```python
from build123d import *

# Parameters (mm, degrees)
SKETCH1_W           = 15
SKETCH1_H           = 35
SKETCH1_W_2         = 1.272906456
SKETCH1_H_2         = 13.426112712
SKETCH1_R           = 1.6
BOSS_EXTRUDE4_DEPTH = 10
SKETCH1_9_R         = 2.4
SKETCH1_9_R_2       = 1.6
CUT_EXTRUDE3_DEPTH  = 8
SKETCH1_10_W        = 15
SKETCH1_10_H        = 5
SKETCH1_10_W_2      = 5
BOSS_EXTRUDE5_DEPTH = 13
BOSS_EXTRUDE6_START = 13
SKETCH1_11_W        = 5
SKETCH1_11_H        = 5
SKETCH1_11_W_2      = 15
BOSS_EXTRUDE6_DEPTH = 10


with BuildPart() as part:
    # Sketch1 → Boss-Extrude4 (new body)
    with BuildSketch(Plane.XY):
        Rectangle(SKETCH1_W, SKETCH1_H)
        with Locations((0, 9.851749103)):
            Rectangle(SKETCH1_W_2, SKETCH1_H_2, mode=Mode.SUBTRACT)
        Circle(SKETCH1_R, mode=Mode.SUBTRACT)
    extrude(amount=BOSS_EXTRUDE4_DEPTH)

    # Sketch1_9 → Cut-Extrude3 (cut)
    with BuildSketch(Plane.XY):
        Circle(SKETCH1_9_R)
        Circle(SKETCH1_9_R_2, mode=Mode.SUBTRACT)
    extrude(amount=CUT_EXTRUDE3_DEPTH, mode=Mode.SUBTRACT)

    # Sketch1_10 → Boss-Extrude5 (add)
    with BuildSketch(Plane.XY):
        with Locations((0, -15)):
            Rectangle(SKETCH1_10_W, SKETCH1_10_H)
        with Locations((-5, 15)):
            Rectangle(SKETCH1_10_W_2, SKETCH1_10_H)
        with Locations((5, 15)):
            Rectangle(SKETCH1_10_W_2, SKETCH1_10_H)
    extrude(amount=BOSS_EXTRUDE5_DEPTH)

    # Sketch1_11 → Boss-Extrude6 (add)
    # profile 1 of 4: a face of its own
    with BuildSketch(Plane.XY.offset(BOSS_EXTRUDE6_START)):
        Polygon((-7.5, 12.5), (-7.5, -12.5), (7.5, -12.5), (7.5, 12.5), (2.5, 12.5), (2.5, 17.5), (-2.5, 17.5), (-2.5, 12.5), align=None)
        with BuildLine():
            Line((-0.636453228, 16.564805459), (0.636453228, 16.564805459))
            Line((0.636453228, 16.564805459), (0.636453228, 4.959327302))
            ThreePointArc((0.636453228, 4.959327302), (3.753815801, 3.302857389), (5, 0))
            ThreePointArc((5, 0), (-3.302857389, -3.753815801), (-0.636453228, 4.959327302))
            Line((-0.636453228, 4.959327302), (-0.636453228, 16.564805459))
        make_face(mode=Mode.SUBTRACT)
    # profile 2 of 4: a face of its own
    with BuildSketch(Plane.XY.offset(BOSS_EXTRUDE6_START)):
        with Locations((-5, 15)):
            Rectangle(SKETCH1_11_W, SKETCH1_11_H)
    # profile 3 of 4: a face of its own
    with BuildSketch(Plane.XY.offset(BOSS_EXTRUDE6_START)):
        with Locations((5, 15)):
            Rectangle(SKETCH1_11_W, SKETCH1_11_H)
    # profile 4 of 4: a face of its own
    with BuildSketch(Plane.XY.offset(BOSS_EXTRUDE6_START)):
        with Locations((0, -15)):
            Rectangle(SKETCH1_11_W_2, SKETCH1_11_H)
    extrude(amount=BOSS_EXTRUDE6_DEPTH)


solid = part.part
```
The model under review builds one solid part; all positions refer to its coordinate system, in mm. A direction names the side the tool comes from. Give positions to 0.01 mm unless a question says otherwise; leave off trailing zeros. Write each loop counter-clockwise with the first axis right and the second up, starting at its lowest first coordinate (ties: lowest second). Pieces come first, ordered by that corner, then holes. Notation, with made-up numbers: (-37.75, 17.25) -> (2.25, 17.25) arc R25 ccw to (2.25, 36.25) -> close; hole circle Ø9 at (17.25, -20). An arc over 180 degrees is marked (long way). Put each result on its own line as item: value.
(1) We need section C-C, the plane y = -9. Give the boundary of the cut face in (x, z), and give its area (3 significant figures).
Results are:
outline: (-7.5, 0) -> (7.5, 0) -> (7.5, 10) -> (-7.5, 10) -> close; (-7.5, 13) -> (7.5, 13) -> (7.5, 23) -> (-7.5, 23) -> close
area: 300 mm²
(2) We need section A-A, the plane x = 0. Give the boundary of the cut face in (y, z), and give its area (3 significant figures).
Results are:
outline: (-17.5, 0) -> (-2.4, 0) -> (-2.4, 8) -> (-1.6, 8) -> (-1.6, 10) -> (-12.5, 10) -> (-12.5, 13) -> (-5, 13) -> (-5, 23) -> (-17.5, 23) -> close; (1.6, 8) -> (2.4, 8) -> (2.4, 0) -> (3.14, 0) -> (3.14, 10) -> (1.6, 10) -> close; (16.56, 0) -> (17.5, 0) -> (17.5, 10) -> (16.56, 10) -> close; (16.56, 13) -> (17.5, 13) -> (17.5, 23) -> (16.56, 23) -> close
area: 320 mm²
(3) We need section D-D, the plane x = 5.5. Give the boundary of the cut face in (y, z), and give its area (3 significant figures).
Results are:
outline: (-17.5, 0) -> (17.5, 0) -> (17.5, 23) -> (-17.5, 23) -> close; hole (-12.5, 10) -> (12.5, 10) -> (12.5, 13) -> (-12.5, 13) -> close
area: 730 mm²
(4) Tool access review of faces 1 (the cylindrical face through (1.29, 2.024, 3.944)), 2 (the flat face through (-0.636, 10, 5)), 3 (the flat face through (2.5, 15, 11)), 4 (the flat face through (5, 12.5, 11)): name each direction out of +Z, -Z, +X, -X, +Y, -Y from which nothing blocks a thin tool from reaching the whole face with its end or side.
Results are:
face 1: -Z
face 2: +Z, -Z
face 3: +Y
face 4: +X, -X
(5) To check wall thickness, follow probe 1 along Y at (x, z) = (0, 9.2); probe 2 along Y at (x, z) = (0, 3); probe 3 along Y at (x, z) = (0, 19.5). State the ranges of each line that lie inside material, in increasing order. Write a range as from..to.
Results are:
probe 1: -17.5..-1.6, 1.6..3.14, 16.56..17.5
probe 2: -17.5..-2.4, 2.4..3.14, 16.56..17.5
probe 3: -17.5..-5, 16.56..17.5
(6) The part is to be moulded in two halves that separate along Z. For faces 5 (the flat face through (-3.4, 4.1, 23)), 6 (the flat face through (0, -2, 8)), 7 (the flat face through (-2, -1, 10)), say which applies: pulls with the +Z half, pulls with the -Z half, needs draft (parallel to the pull), parting line crosses it, or undercut.
Results are:
face 5: pulls with the +Z half
face 6: pulls with the -Z half
face 7: undercut
(7) We need section B-B, the plane z = 11.25. Give the boundary of the cut face in (x, y), and give its area (3 significant figures).
Results are:
outline: (-7.5, -17.5) -> (7.5, -17.5) -> (7.5, -12.5) -> (-7.5, -12.5) -> close; (-7.5, 12.5) -> (-2.5, 12.5) -> (-2.5, 17.5) -> (-7.5, 17.5) -> close; (2.5, 12.5) -> (7.5, 12.5) -> (7.5, 17.5) -> (2.5, 17.5) -> close
area: 125 mm²
(8) For pin 1 Ø9 at (x, y) = (0, 0) entering from +Z, flat-tipped, find the tip position at first contact; note if it passes through.
Results are:
pin 1: z = 10
